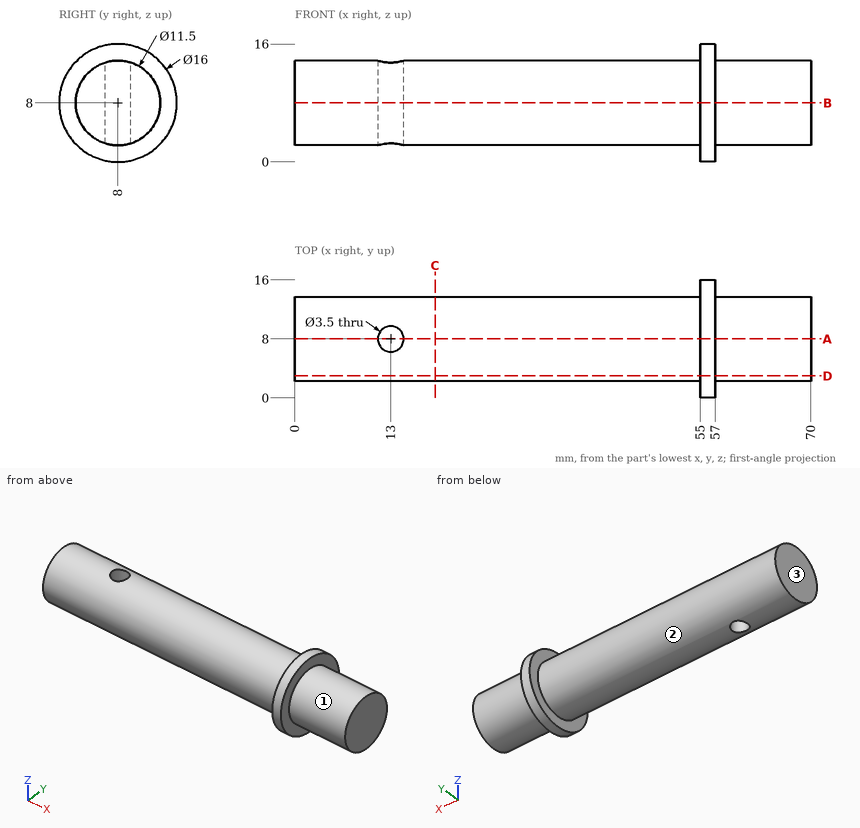
Source: three-view drawing plus pictorial views. Frame: mm from the lowest corner of the part. A direction names the side the tool comes from. Give positions to 0.01 mm unless a question says otherwise; leave off trailing zeros. Write each loop counter-clockwise with the first axis right and the second up, starting at its lowest first coordinate (ties: lowest second). Pieces come first, ordered by that corner, then holes. Notation, with made-up numbers: (76, -19.5) -> (114, -19.5) arc R30 cw to (114, 17.5) -> close; hole circle Ø5 at (88, 84). An arc over 180 degrees is marked (long way). Answer in a Markdown table with one row per item.
(1) Section query B-B on z = 8. Return loops of the section in (x, y).
Answers below:
| item | result |
|---|---|
| outline | (0, 2.25) -> (55, 2.25) -> (55, 0) -> (57, 0) -> (57, 2.25) -> (70, 2.25) -> (70, 13.75) -> (57, 13.75) -> (57, 16) -> (55, 16) -> (55, 13.75) -> (0, 13.75) -> close; hole circle Ø3.5 at (13, 8) |
(2) Section query D-D on y = 3. Return loops of the section in (x, z) (3 decimals), then the cut area to 3 significant figures.
Answers below:
| item | result |
|---|---|
| outline | (0, 5.161) -> (55, 5.161) -> (55, 1.755) -> (57, 1.755) -> (57, 5.161) -> (70, 5.161) -> (70, 10.839) -> (57, 10.839) -> (57, 14.245) -> (55, 14.245) -> (55, 10.839) -> (0, 10.839) -> close |
| area | 411 mm^2 |
(3) Pin query (flat end, axial travel): pin 1 (5 mm diameter, centred on x = 20, y = 8.5, fed in from -Z); pin 2 (2 mm diameter, centred on x = 13, y = 8, fed in from +Z); pin 3 (8 mm diameter, centred on x = 29, y = 9, fed in from +Z); pin 4 (2 mm diameter, centred on y = 2, z = 13.5, fed in from -X). Return the tip coordinate at first contact, or that it passes through.
Answers below:
| item | result |
|---|---|
| pin 1 | z = 2.25 |
| pin 2 | through |
| pin 3 | z = 13.75 |
| pin 4 | x = 55 |
(4) Ray query, line 1 along X through (y, z) = (8, 10.5); line 2 along X through (y, z) = (7, 15); line 3 along Y through (x, z) = (13, 5). Return the intervals inside material, ascending. Write a range as [from, to].
Answers below:
| item | result |
|---|---|
| line 1 | [0, 11.25], [14.75, 70] |
| line 2 | [55, 57] |
| line 3 | [3.09, 6.25], [9.75, 12.91] |
(5) Section query C-C on x = 19. Return loops of the section in (y, z), then the cut area to 3 significant figures.
Answers below:
| item | result |
|---|---|
| outline | circle Ø11.5 at (8, 8) |
| area | 104 mm^2 |
(6) Section query A-A on y = 8. Return loops of the section in (x, z).
Answers below:
| item | result |
|---|---|
| outline | (0, 2.25) -> (11.25, 2.25) -> (11.25, 13.75) -> (0, 13.75) -> close; (14.75, 2.25) -> (55, 2.25) -> (55, 0) -> (57, 0) -> (57, 2.25) -> (70, 2.25) -> (70, 13.75) -> (57, 13.75) -> (57, 16) -> (55, 16) -> (55, 13.75) -> (14.75, 13.75) -> close |
(7) Set-up query: the marked faces 1, 2 and 3. Return all of +Z, -Z, +X, -X, +Y, -Y with unobstructed straight access to the full face (end or side cutting, diameter ignored); none if empty.
Answers below:
| item | result |
|---|---|
| face 1 | +X |
| face 2 | -X |
| face 3 | +Z, -Z, -X, +Y, -Y |
